Source: CAD feature listing. Evaluate the final solid. Frame: model axes, mm. Face numbers are marked on the shaded views. Give positions to 0.01 mm unless a question says otherwise; leave off trailing zeros. Loops run counter-clockwise (first coordinate to the right, second up) from the corner with the lowest first, then second, coordinate; pieces in that order, holes last. Notation, with made-up numbers: (-29, 7) -> (-12, 7) arc R15 cw to (-12, 20) -> close; hole circle Ø9 at (17, -30.75). An arc over 180 degrees is marked (long way). Return JSON: item names as keys, results as strings. Group by question number.
```python
from build123d import *

# Parameters (mm, degrees)
F1_DEPTH = 1.75
F2_T     = 1


with BuildPart() as f1:
    # F0 (on Top) → F1 (new body)
    with BuildSketch(Plane.XY):
        Polygon((39.8734986782, 16), (39.8734986782, -16), (64.8734986782, -16), (64.8734986782, 12), (60.8734986782, 16), align=None)
    extrude(amount=F1_DEPTH)

    # F2
    f2_openings = [f1.faces().sort_by_distance(p)[0] for p in [
        (52.260704, -0.148148, 1.75),
    ]]
    offset(amount=F2_T, openings=f2_openings, kind=Kind.INTERSECTION)


solid = f1.part
```
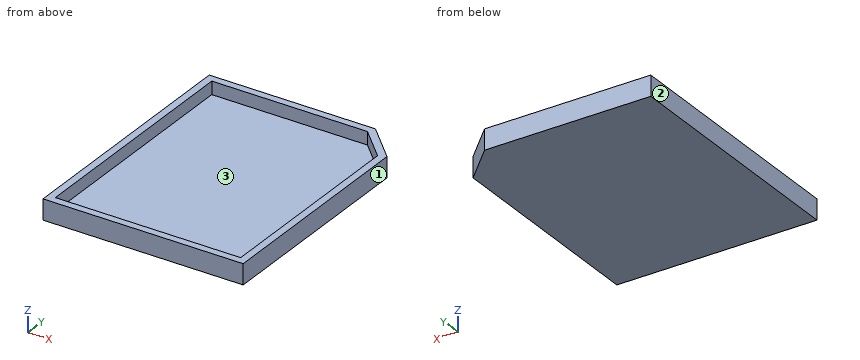
1) Cut plane A-A on z = 1.2. Return loops of the section in (x, y).
2) Cut plane C-C on x = 45.5. Return loops of the section in (y, z), then the cut area to 3 significant figures.
3) Material intervals for line 1 (Y direction, x = 45, z = 0.8); line 2 (X direction, y = 1, z = 0.1); line 3 (Z direction, x = 51.5, y = -11), sorted ascending.
4) Cut plane B-B on y = 9. Return loops of the section in (x, z).
5) Mould query, pull axis X, two halves, no side actions, for the marked faces 1, 2 and 3. Classes: released by +X, released by -X, zero draft, split by the parting line, or undercut.
6) Contact query for a flat-ended pin moving along its axis: P1, Ø12, axis at x = 46.5, y = 0.5, coming from the +Z side. Output: stop coordinate, or through.
Calculated:
{
 "1": {"outline": "(38.87, -17) -> (65.87, -17) -> (65.87, 12.41) -> (61.29, 17) -> (38.87, 17) -> close; hole (39.87, -16) -> (64.87, -16) -> (64.87, 12) -> (60.87, 16) -> (39.87, 16) -> close"},
 "2": {"outline": "(-17, -1) -> (17, -1) -> (17, 1.75) -> (16, 1.75) -> (16, 0) -> (-16, 0) -> (-16, 1.75) -> (-17, 1.75) -> close", "area": "37.5 mm2"},
 "3": {"line 1": "-17 to -16, 16 to 17", "line 2": "38.87 to 39.87, 64.87 to 65.87", "line 3": "-1 to 0"},
 "4": {"outline": "(38.87, -1) -> (65.87, -1) -> (65.87, 1.75) -> (64.87, 1.75) -> (64.87, 0) -> (39.87, 0) -> (39.87, 1.75) -> (38.87, 1.75) -> close"},
 "5": {"face 1": "released by +X", "face 2": "released by -X", "face 3": "undercut"},
 "6": {"P1": "z = 0"}
}
